Here's how the part is built. I have some questions about the finished solid (model axes, mm). A direction names the side the tool comes from. Round coordinates to 2 decimals unless told otherwise and drop trailing zeros. Loops run counter-clockwise (first coordinate to the right, second up) from the corner with the lowest first, then second, coordinate; pieces in that order, holes last. Notation, with made-up numbers: (30, 69) -> (38, 69) arc R18 ccw to (38, 93) -> close; hole circle Ø10 at (42, 47.5). An arc over 180 degrees is marked (long way). Use one line per item in the form item = value. Start each with the question number.
Item 1: If I drill on L1, parallel to Y at x = 120, z = 0.5; L2, parallel to Z at x = 58.5, y = 6; L3, parallel to Y at x = 0, z = 1.25, over which ranges is the centre line in solid material (lowest first)? Write a range as [from, to].
Item 2: If we section it at B-B (y = 0): Write out the boundary of the cut face in (x, z).
Item 3: Thinking about a two-plate mould opening in Y: for faces 1 (the face through (134, 0, 0)), 2 (the face through (40, 0, 0)), 3 (the face through (107.753, -0.517, -0.035)), 4 (the face through (59, 14, 2)), which applies, released by +Y, released by -Y, zero draft, split by the parting line, or undercut?
Item 4: If we section it at A-A (x = 109): Write out the boundary of the cut face in (y, z).
Item 5: I'm going to push flat-ended pins straight in: pin 1 Ø1.6 at (x, y) = (112.22, -7.78) entering from +Z; pin 2 Ø0.8 at (y, z) = (-5.5, -0.5) entering from -X; pin 3 Ø11.5 at (x, y) = (120, 0) entering from +Z; pin 4 Ø2 at (y, z) = (-3, 4) entering from +X. Where does each tip first touch, or does it pass through?
Item 6: If we section it at D-D (x = 131): Write out the boundary of the cut face in (y, z).
Item 7: If we section it at C-C (y = 11): Write out the boundary of the cut face in (x, z), then the cut area to 3 significant figures.
Item 8: For faces 5 (the face through (114, 0, 2.5)), 6 (the face through (96, 0, -1)), 7 (the face through (110.934, -7.373, -0.035)), which set-ups out of +Z, -Z, +X, -X, +Y, -Y let a thin tool reach every point of the face, with its end or its side?
```python
from build123d import *

# Parameters (mm, degrees)
RESSALTO_EXTRUS_O1_DEPTH = 5
ESBO_O2_R                = 1.35
ESBO_O2_R_2              = 1.373066436
ESBO_O2_R_3              = 1.330065432
ESBO_O2_R_4              = 5
CORTE_EXTRUS_O1_DEPTH    = 137.810087347
ESBO_O3_R                = 5
CORTE_EXTRUS_O2_DEPTH    = 137.810087347
ESBO_O5_W                = 31.24115408
ESBO_O5_H                = 28
CORTE_EXTRUS_O3_DEPTH    = 137.810087347
ESBO_O6_W                = 5
ESBO_O6_H                = 28
RESSALTO_EXTRUS_O2_DEPTH = 2.5
RESSALTO_EXTRUS_O4_DEPTH = 5
ESBO_O8_R                = 5
ESBO_O8_R_2              = 1.35
CORTE_EXTRUS_O4_DEPTH    = 135.937948702
ESBO_O10_W               = 5
ESBO_O10_H               = 2.5
CORTE_EXTRUS_O5_DEPTH    = 137.985400682
ESBO_O11_W               = 5
ESBO_O11_H               = 2.5
RESSALTO_EXTRUS_O5_DEPTH = 28


with BuildPart() as part:
    # Esboço1 → Ressalto-extrusão1 (new body)
    with BuildSketch(Plane.XY):
        with BuildLine():
            Line((0, -14), (122, -14))
            ThreePointArc((122, -14), (136, 0), (122, 14))
            Line((122, 14), (0, 14))
            ThreePointArc((0, 14), (-14, 0), (0, -14))
        make_face()
    extrude(amount=RESSALTO_EXTRUS_O1_DEPTH)

    # Esboço2 → Corte-extrusão1 (cut, through all)
    with BuildSketch(Plane(origin=(0, 0, 0), x_dir=(-1, 0, 0), z_dir=(0, 0, -1))):
        with Locations((-125.327123404, 10.484762747)):
            Circle(ESBO_O2_R)
        with Locations((-116.938784683, 9.766478358)):
            Circle(ESBO_O2_R)
        with Locations((-111.515237253, 3.327123404)):
            Circle(ESBO_O2_R)
        with Locations((-112.233521642, -5.061215317)):
            Circle(ESBO_O2_R)
        with Locations((-118.672876596, -10.484762747)):
            Circle(ESBO_O2_R_2)
        with Locations((-127.061215317, -9.766478358)):
            Circle(ESBO_O2_R_3)
        with Locations((-132.484762747, -3.327123404)):
            Circle(ESBO_O2_R)
        with Locations((-131.766478358, 5.061215317)):
            Circle(ESBO_O2_R)
        with Locations((-122, 0)):
            Circle(ESBO_O2_R_4)
    extrude(amount=-CORTE_EXTRUS_O1_DEPTH, mode=Mode.SUBTRACT)

    # Esboço3 → Corte-extrusão2 (cut, through all)
    with BuildSketch(Plane(origin=(0, 0, 0), x_dir=(-1, 0, 0), z_dir=(0, 0, -1))):
        Circle(ESBO_O3_R)
    extrude(amount=-CORTE_EXTRUS_O2_DEPTH, mode=Mode.SUBTRACT)

    # Esboço5 → Corte-extrusão3 (cut, through all)
    with BuildSketch(Plane(origin=(0, 0, 0), x_dir=(-1, 0, 0), z_dir=(0, 0, -1))):
        with Locations((-121.62057704, 0)):
            Rectangle(ESBO_O5_W, ESBO_O5_H)
    extrude(amount=-CORTE_EXTRUS_O3_DEPTH, mode=Mode.SUBTRACT)

    # Esboço6 → Ressalto-extrusão2 (add)
    with BuildSketch(Plane(origin=(0, 0, 0), x_dir=(-1, 0, 0), z_dir=(0, 0, -1))):
        with Locations((-103.5, 0)):
            Rectangle(ESBO_O6_W, ESBO_O6_H)
    extrude(amount=RESSALTO_EXTRUS_O2_DEPTH)

    # Esboço7 → Ressalto-extrusão4 (add)
    with BuildSketch(Plane(origin=(0, 0, -2.5), x_dir=(-1, 0, 0), z_dir=(0, 0, -1))):
        with BuildLine():
            Line((-106, 14), (-120, 14))
            ThreePointArc((-120, 14), (-134, 0), (-120, -14))
            Line((-120, -14), (-106, -14))
            Line((-106, -14), (-106, 14))
        make_face()
    extrude(amount=-RESSALTO_EXTRUS_O4_DEPTH)

    # Esboço8 → Corte-extrusão4 (cut, through all)
    with BuildSketch(Plane(origin=(0, 0, -2.5), x_dir=(-1, 0, 0), z_dir=(0, 0, -1))):
        with Locations((-120, 0)):
            Circle(ESBO_O8_R)
        with Locations((-120, 11)):
            Circle(ESBO_O8_R_2)
        with Locations((-109, 0)):
            Circle(ESBO_O8_R_2)
        with Locations((-120, -11)):
            Circle(ESBO_O8_R_2)
        with Locations((-131, 0)):
            Circle(ESBO_O8_R_2)
        with Locations((-112.221825407, 7.778174593)):
            Circle(ESBO_O8_R_2)
        with Locations((-112.221825407, -7.778174593)):
            Circle(ESBO_O8_R_2)
        with Locations((-127.778174593, -7.778174593)):
            Circle(ESBO_O8_R_2)
        with Locations((-127.778174593, 7.778174593)):
            Circle(ESBO_O8_R_2)
    extrude(amount=-CORTE_EXTRUS_O4_DEPTH, mode=Mode.SUBTRACT)

    # Esboço10 → Corte-extrusão5 (cut, through all)
    with BuildSketch(Plane.XZ.offset(14)):
        with Locations((103.5, 3.75)):
            Rectangle(ESBO_O10_W, ESBO_O10_H)
    extrude(amount=-CORTE_EXTRUS_O5_DEPTH, mode=Mode.SUBTRACT)

    # Esboço11 → Ressalto-extrusão5 (add, through all)
    with BuildSketch(Plane.XZ.offset(14)):
        with Locations((98.5, -1.25)):
            Rectangle(ESBO_O11_W, ESBO_O11_H)
    extrude(amount=-RESSALTO_EXTRUS_O5_DEPTH)


solid = part.part
```
Values found:
q1.L1 = [-14, -12.35], [-9.65, -5], [5, 9.65], [12.35, 14]
q1.L2 = [0, 5]
q1.L3 = [-14, -5], [5, 14]
q2.outline = (-14, 0) -> (-5, 0) -> (-5, 5) -> (-14, 5) -> close; (5, 0) -> (96, 0) -> (96, -2.5) -> (107.65, -2.5) -> (107.65, 2.5) -> (101, 2.5) -> (101, 5) -> (5, 5) -> close; (110.35, -2.5) -> (115, -2.5) -> (115, 2.5) -> (110.35, 2.5) -> close; (125, -2.5) -> (129.65, -2.5) -> (129.65, 2.5) -> (125, 2.5) -> close; (132.35, -2.5) -> (134, -2.5) -> (134, 2.5) -> (132.35, 2.5) -> close
q3.face_1 = split by the parting line
q3.face_2 = zero draft
q3.face_3 = undercut
q3.face_4 = released by +Y
q4.outline = (-14, -2.5) -> (-1.35, -2.5) -> (-1.35, 2.5) -> (-14, 2.5) -> close; (1.35, -2.5) -> (14, -2.5) -> (14, 2.5) -> (1.35, 2.5) -> close
q5.pin_1 = through
q5.pin_2 = 96
q5.pin_3 = 2.5
q5.pin_4 = 101
q6.outline = (-8.66, -2.5) -> (-1.35, -2.5) -> (-1.35, 2.5) -> (-8.66, 2.5) -> close; (1.35, -2.5) -> (8.66, -2.5) -> (8.66, 2.5) -> (1.35, 2.5) -> close
q7.outline = (-8.66, 0) -> (96, 0) -> (96, -2.5) -> (118.65, -2.5) -> (118.65, 2.5) -> (101, 2.5) -> (101, 5) -> (-8.66, 5) -> close; (121.35, -2.5) -> (128.66, -2.5) -> (128.66, 2.5) -> (121.35, 2.5) -> close
q7.area = 686 mm2
q8.face_5 = +Z, +X, +Y, -Y
q8.face_6 = -Z, -X, +Y, -Y
q8.face_7 = +Z, -Z
